Could you check a few things on this model? Use its own coordinates, in mm. A direction names the side the tool comes from. Coordinates: 2 decimals unless noted, no trailing zeros. Order: outer loops, then holes, each group sorted by start corner. A loop starts at its lowest first (then second) coordinate and runs counter-clockwise, first axis right, second up. Notation, with made-up numbers: (76.5, 76) -> (96.5, 76) arc R23 ccw to (96.5, 113) -> close; hole circle Ø2 at (7, 48). An arc over 180 degrees is marked (long way). Return JSON: item names as keys, results as strings. Group by question number.
from build123d import *

# Parameters (mm, degrees)
F0_W          = 101.8202751875
F0_H          = 98.3881354332
F0_R          = 25.4
F1_DEPTH      = 101.6
F4_R          = 25.4
F5_DEPTH      = 50.8
F5_DEPTH_BACK = 152.4


# Not quite as in the source:
# - a feature of the source that left no trace in its solid (it failed there, or was rolled back) is left out


with BuildPart() as f1:
    # F0 (on Front) → F1 (new body)
    with BuildSketch(Plane.XZ):
        with Locations((50.9101375937, 49.1940677166)):
            Rectangle(F0_W, F0_H)
        with Locations((50.9101375937, 49.1940677166)):
            Circle(F0_R, mode=Mode.SUBTRACT)
    extrude(amount=F1_DEPTH)

    # F4 (on offset) → F5 (join, two sides)
    with BuildSketch(Plane.XZ.offset(101.6)) as f5_sk:
        Circle(F4_R)
    extrude(amount=F5_DEPTH)
    extrude(f5_sk.sketch, amount=-F5_DEPTH_BACK)


solid = f1.part
Q1. I want a section at A-A on z = 55.5. Please give me the cut outline in (x, y).
Q2. I'm going to push flat-ended pins straight in: pin 1 Ø5 at (x, z) = (36.5, 14.5) entering from +Y; pin 2 Ø10 at (y, z) = (-52.5, 70) entering from -X; pin 3 Ø10 at (x, y) = (-6.5, 28.5) entering from +Z. Where does each tip first touch, or does it pass through?
Q3. I want a section at D-D on z = 11.5. Please give me the cut outline in (x, y), and give its area (3 significant figures).
Q4. I need wall thicknesses on line 1 along Y through (x, z) = (36, 80); line 2 along X through (y, z) = (-63.5, 86.5); line 3 along Z through (x, y) = (64.5, -3). Which ranges of each line are inside material? Lowest first, please. Write a range as from..to.
Q5. On a 3-axis mill with a long thin cutter (end or side, diameter ignored), from which of +Z, -Z, +X, -X, +Y, -Y can I reach the whole of each face in a straight line? I mean faces 1 (the flat face through (101.82, -50, 49)), 2 (the flat face through (0, -50, 61)), 3 (the flat face through (39, -101.6, 72)). Say none if no direction works.
Q6. We'd pull the mould along Z, two halves only. Please class faces 4 (the cylindrical face through (62.63, -50.09, 26.66)), 5 (the flat face through (39, 0, 72)), 6 (the flat face through (50, -50, 98.388)), 7 (the flat face through (63, -50, 0)): pulls with the +Z half, pulls with the -Z half, needs draft (parallel to the pull), parting line crosses it, or undercut.
Q7. I want a section at C-C on y = -44.5. Please give me the cut outline in (x, z), and give its area (3 significant figures).
Q8. I want a section at B-B on x = 46. Please give me the cut outline in (y, z), and give its area (3 significant figures).
Response values:
{
 "1": {"outline": "(0, -101.6) -> (26.31, -101.6) -> (26.31, 0) -> (0, 0) -> close; (75.51, -101.6) -> (101.82, -101.6) -> (101.82, 0) -> (75.51, 0) -> close"},
 "2": {"pin 1": "stops at y = 0", "pin 2": "stops at x = 0", "pin 3": "stops at z = 25.36"},
 "3": {"outline": "(-22.65, -152.4) -> (22.65, -152.4) -> (22.65, -101.6) -> (101.82, -101.6) -> (101.82, 0) -> (22.65, 0) -> (22.65, 50.8) -> (-22.65, 50.8) -> close", "area": "17,200 mm²"},
 "4": {"line 1": "y = -101.6..0", "line 2": "x = 0..101.82", "line 3": "z = 0..27.74, 70.65..98.39"},
 "5": {"face 1": "+Z, -Z, +X, +Y, -Y", "face 2": "+Z, -X, +Y, -Y", "face 3": "+Z, +X, -Y"},
 "6": {"face 4": "undercut", "face 5": "needs draft", "face 6": "pulls with the +Z half", "face 7": "pulls with the -Z half"},
 "7": {"outline": "(0, 25.4) arc R25.4 ccw (long way) to (25.4, 0) -> (101.82, 0) -> (101.82, 98.39) -> (0, 98.39) -> close; hole circle Ø50.8 at (50.91, 49.19)", "area": "9,510 mm²"},
 "8": {"outline": "(-101.6, 0) -> (0, 0) -> (0, 24.27) -> (-101.6, 24.27) -> close; (-101.6, 74.11) -> (0, 74.11) -> (0, 98.39) -> (-101.6, 98.39) -> close", "area": "4,930 mm²"}
}
